```python
from build123d import *

# Parameters (mm, degrees)
ESBO_O1_R                = 55
RESSALTO_EXTRUS_O1_DEPTH = 25
ESBO_O2_R                = 50
RESSALTO_EXTRUS_O2_DEPTH = 10
CASCA1_T                 = -5
FILETE2_R                = 2
FILETE3_R                = 2


with BuildPart() as part:
    # Esboço1 → Ressalto-extrusão1 (new body)
    with BuildSketch(Plane.XY):
        Circle(ESBO_O1_R)
    extrude(amount=RESSALTO_EXTRUS_O1_DEPTH)

    # Esboço2 → Ressalto-extrusão2 (add)
    with BuildSketch(Plane(origin=(0, 0, 0), x_dir=(-1, 0, 0), z_dir=(0, 0, -1))):
        Circle(ESBO_O2_R)
    extrude(amount=RESSALTO_EXTRUS_O2_DEPTH)

    # Casca1
    casca1_openings = [part.faces().sort_by_distance(p)[0] for p in [
        (0, 0, 25),
    ]]
    offset(amount=CASCA1_T, openings=casca1_openings, kind=Kind.INTERSECTION)

    # Filete2
    filete2_edges = [part.edges().sort_by_distance(p)[0] for p in [
        (50, 0, 0),
        (50, 0, -10),
    ]]
    fillet(filete2_edges, radius=FILETE2_R)

    # Filete3
    filete3_edges = [part.edges().sort_by_distance(p)[0] for p in [
        (-55, 0, 0),
    ]]
    fillet(filete3_edges, radius=FILETE3_R)


solid = part.part
```
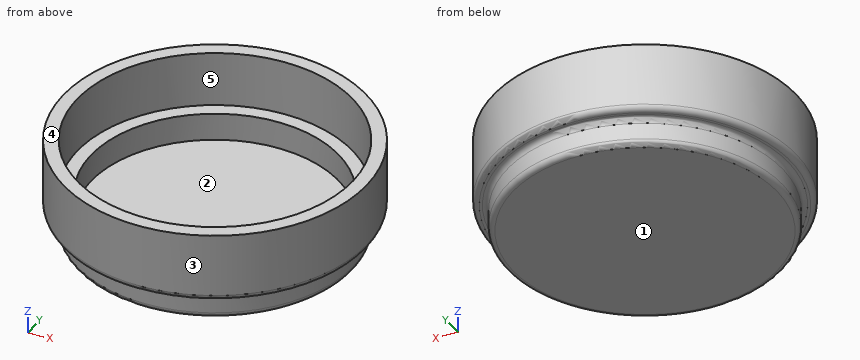
Geometry check sheet. Reference: the model listing, model coordinates, mm. Face numbers are marked on the shaded views. A direction names the side the tool comes from. Coordinates: 2 decimals unless noted, no trailing zeros. Order: outer loops, then holes, each group sorted by start corner. A loop starts at its lowest first (then second) coordinate and runs counter-clockwise, first axis right, second up.
Item 1: Scan lines: line 1 along Y through (x, z) = (0, 15); line 2 along Y through (x, z) = (0, 2); line 3 along X through (y, z) = (43, 5.5). Record each from-to range of solid material in increasing order.
Item 2: Depth check by flat-ended pin: pin 1 (3 mm diameter, centred on x = 32, z = 0.5, fed in from -Y); pin 2 (5 mm diameter, centred on x = -7.5, z = -4.5, fed in from -Y); pin 3 (1 mm diameter, centred on x = -1.5, z = 12, fed in from -Y). Enter the tip coordinate at first touch or a pass-through.
Item 3: Tool access check on the marked faces 1 and 2. Record the directions out of +Z, -Z, +X, -X, +Y, -Y that give a thin tool (end or side, any length) a straight path to the whole face; none if there is none.
Item 4: Mould release check, pull along X, two halves, no side actions. Record for the marked faces 3, 4 and 5: released by +X, released by -X, zero draft, split by the parting line, or undercut.
Item 5: Section check C-C (z = 11.5). Enter the section's corners in (x, y).
Item 6: Section check A-A (y = 0). Enter the section's corners in (x, z), plus the area to 3 significant figures.
Check sheet entries:
1. line 1: y = -55 to -50, 50 to 55
1. line 2: y = -55 to -45, 45 to 55
1. line 3: x = -34.29 to -25.51, 25.51 to 34.29
2. pin 1: stops at y = -45.46
2. pin 2: stops at y = -49.75
2. pin 3: stops at y = -54.99
3. face 1: -Z, +X, -X, +Y, -Y
3. face 2: +Z
4. face 3: split by the parting line
4. face 4: zero draft
4. face 5: undercut
5. outline: circle Ø110 at (0, 0); hole circle Ø100 at (0, 0)
6. outline: (-55, 2) arc R2 ccw to (-53, 0) - (-52, 0) arc R2 cw to (-50, -2) - (-50, -8) arc R2 ccw to (-48, -10) - (48, -10) arc R2 ccw to (50, -8) - (50, -2) arc R2 cw to (52, 0) - (53, 0) arc R2 ccw to (55, 2) - (55, 25) - (50, 25) - (50, 5) - (45, 5) - (45, -5) - (-45, -5) - (-45, 5) - (-50, 5) - (-50, 25) - (-55, 25) - close
6. area: 848 mm2
